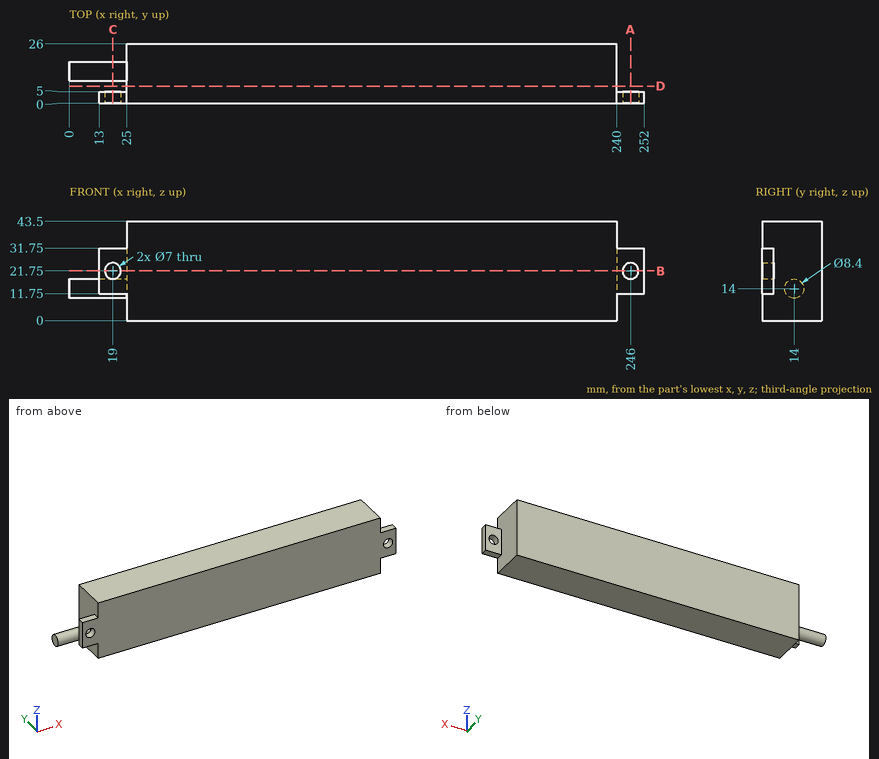
Here's the drawing with two shaded views (mm, measured from the low corner). I have some questions. Coordinates: 2 decimals unless noted, no trailing zeros. Loops run counter-clockwise (first coordinate to the right, second up) from the corner with the lowest first, then second, coordinate; pieces in that order, holes last. Notation, with made-up numbers: M 49,39 L 79,39 A28 cw 79,73 Z; hole C -20.75,84 d1. An arc over 180 degrees is marked long. Put each result on its own line as item: value. Start each with the question number.
(1) Will these pins go through, and if not, where does the flat tip stop? pin 1 Ø2.5 at (x, y) = (243, 3.5) entering from -Z; pin 2 Ø2.5 at (y, z) = (1.5, 24) entering from -X; pin 3 Ø4 at (x, z) = (246, 21.75) entering from +Y; pin 4 Ø6 at (y, z) = (6, 6) entering from -X.
(2) Imagine slicing it at C-C on x = 19. List the corners of the cut face in (y, z) for me, and give its area (3 significant figures).
(3) I need wall thicknesses on probe 1 along X at (y, z) = (2.15, 21.75); probe 2 along Z at (x, y) = (19, 2.3); probe 3 along X at (y, z) = (2.75, 41.5). Which ranges of each line are inside material? Lowest first, please.
(4) Imagine slicing it at D-D on y = 7.5. List the corners of the cut face in (x, z) for me, and give its area (3 significant figures).
(5) Imagine slicing it at B-B on z = 21.75. List the corners of the cut face in (x, y) for me, and give its area (3 significant figures).
(6) Imagine slicing it at A-A on x = 246. List the corners of the cut face in (y, z) for me, and give its area (3 significant figures).
Worked answers:
1. pin 1: stops at z = 11.75
1. pin 2: stops at x = 13
1. pin 3: passes through
1. pin 4: stops at x = 25
2. outline: M 0,11.75 L 5,11.75 L 5,18.25 L 0,18.25 Z; M 0,25.25 L 5,25.25 L 5,31.75 L 0,31.75 Z; C 14,14 d8.4
2. area: 120 mm2
3. probe 1: x = 13 to 15.5, 22.5 to 242.5, 249.5 to 252
3. probe 2: z = 11.75 to 18.25, 25.25 to 31.75
3. probe 3: x = 25 to 240
4. outline: M 25,0 L 240,0 L 240,43.5 L 25,43.5 Z
4. area: 9,350 mm2
5. outline: M 13,0 L 15.5,0 L 15.5,5 L 13,5 Z; M 22.5,0 L 242.5,0 L 242.5,5 L 240,5 L 240,26 L 25,26 L 25,5 L 22.5,5 Z; M 249.5,0 L 252,0 L 252,5 L 249.5,5 Z
5. area: 5,640 mm2
6. outline: M 0,11.75 L 5,11.75 L 5,18.25 L 0,18.25 Z; M 0,25.25 L 5,25.25 L 5,31.75 L 0,31.75 Z
6. area: 65.0 mm2
